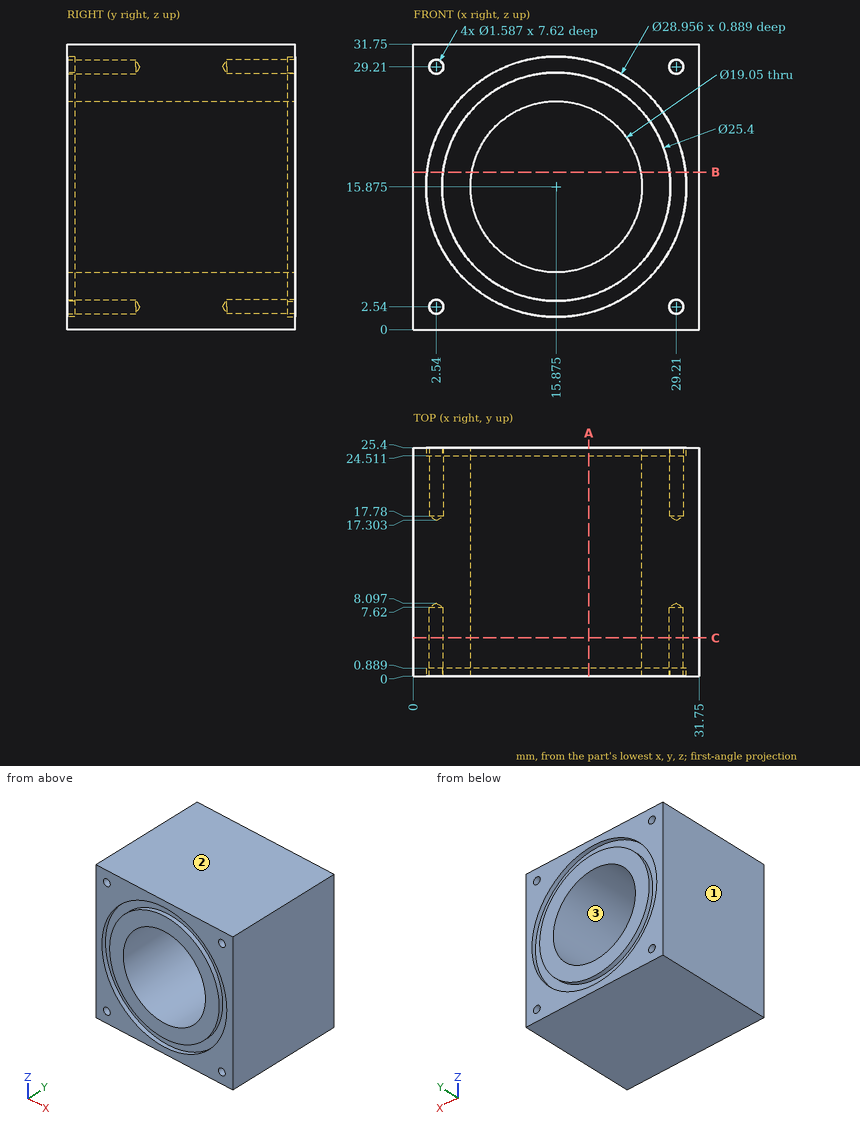
The drawing under review shows one solid part. Ordinate dimensions are in mm from its lowest x, y, z. Give positions to 0.01 mm unless a question says otherwise; leave off trailing zeros. Write each loop counter-clockwise with the first axis right and the second up, starting at its lowest first coordinate (ties: lowest second). Pieces come first, ordered by that corner, then holes. Notation, with made-up numbers: (43.25, -27.5) - (73.25, -27.5) arc R20 cw to (73.25, 1.5) - close; hole circle Ø5 at (-9.5, 29). An arc over 180 degrees is marked (long way). Answer in a Markdown table with one row per item. Add a question column.
1. We need section C-C on y = 4.25. State how many separate pieces and enclosed holes the cut face has, then the cut area to 3 significant figures.
2. Draft analysis for pull direction Z (two halves, no side actions). For the marked faces 1, 2 and 3, state which applies: +Z half, -Z half, draft (parallel to the pull), parting line (faces both ways), or undercut.
3. Insertion check: P1, Ø1, axis at x = 2.54, z = 2.54, coming from the +Y side; P2, Ø8.5, axis at x = 22.5, z = 15.5, coming from the -Y side; P3, Ø1.4, axis at x = 2.54, z = 2.54, coming from the +Y side (1 decimal). Each pin has a flat end and moves straight along its axis. Give the tip position at first contact, or say it passes through.
4. We need section A-A on x = 19.5. Write out the cut boundary in (y, z).
5. Wall thickness on line 1 along X through (y, z) = (6.25, 2.54); line 2 along Y through (x, z) = (3, 17.5): over which ranges is each line inside the solid? List them lowest first. Write a range as [from, to].
6. We need section B-B on z = 17.5. Write out the cut boundary in (x, y).
Ans:
| question | item | result |
|---|---|---|
| 1 | separate pieces | 1 |
| 1 | enclosed holes | 5 |
| 1 | area | 715 mm^2 |
| 2 | face 1 | draft |
| 2 | face 2 | +Z half |
| 2 | face 3 | undercut |
| 3 | P1 | stops at y = 17.6 |
| 3 | P2 | stops at y = 0 |
| 3 | P3 | stops at y = 17.7 |
| 4 | outline | (0, 0) - (25.4, 0) - (25.4, 1.86) - (24.51, 1.86) - (24.51, 3.7) - (25.4, 3.7) - (25.4, 7.07) - (0, 7.07) - (0, 3.7) - (0.89, 3.7) - (0.89, 1.86) - (0, 1.86) - close; (0, 24.68) - (25.4, 24.68) - (25.4, 28.05) - (24.51, 28.05) - (24.51, 29.89) - (25.4, 29.89) - (25.4, 31.75) - (0, 31.75) - (0, 29.89) - (0.89, 29.89) - (0.89, 28.05) - (0, 28.05) - close |
| 5 | line 1 | x = [0, 1.75], [3.33, 28.42], [30, 31.75] |
| 5 | line 2 | y = [0.89, 24.51] |
| 6 | outline | (0, 0) - (1.49, 0) - (1.49, 0.89) - (3.28, 0.89) - (3.28, 0) - (6.49, 0) - (6.49, 25.4) - (3.28, 25.4) - (3.28, 24.51) - (1.49, 24.51) - (1.49, 25.4) - (0, 25.4) - close; (25.26, 0) - (28.47, 0) - (28.47, 0.89) - (30.26, 0.89) - (30.26, 0) - (31.75, 0) - (31.75, 25.4) - (30.26, 25.4) - (30.26, 24.51) - (28.47, 24.51) - (28.47, 25.4) - (25.26, 25.4) - close |
